The listing builds one solid part. Answer for the finished solid, in the listing's coordinates (mm). A direction names the side the tool comes from. Coordinates: 2 decimals unless noted, no trailing zeros. Loops run counter-clockwise (first coordinate to the right, second up) from the corner with the lowest first, then second, coordinate; pieces in that order, holes last. Notation, with made-up numbers: (-26.5, 74.5) - (-20.5, 74.5) arc R19 ccw to (-20.5, 100.5) - close; hole circle Ø6 at (-37, 14). An arc over 180 degrees is marked (long way). Use one line per item in the form item = value. Start each with the question number.
```python
from build123d import *

# Parameters (mm, degrees)
F0_W      = 117.213294
F0_H      = 67.42356
F1_DEPTH  = 25.4
F1_FACE_W = 117.213294
F1_FACE_H = 67.42356
F2_DEPTH  = 12.7
F3_R      = 45.862113
F3_R_2    = 37.681332
F4_DEPTH  = 63.5
F5_W      = 74.026364
F5_H      = 21.373598
F6_DEPTH  = 50.8
F8_DEPTH  = 25.4


with BuildPart() as f1:
    # F0 (on Top) → F1 (new body)
    with BuildSketch(Plane.XY):
        with Locations((9.024359, -5.497601)):
            Rectangle(F0_W, F0_H)
    extrude(amount=F1_DEPTH)

    # F1_face (on face) → F2 (cut)
    with BuildSketch(Plane(origin=(9.024359, -5.497601, 25.4), x_dir=(1, 0, 0), z_dir=(0, 0, 1))):
        Rectangle(F1_FACE_W, F1_FACE_H)
    extrude(amount=-F2_DEPTH, mode=Mode.SUBTRACT)

    # F3 (on Top) → F4 (join)
    with BuildSketch(Plane.XY):
        with Locations((96.162871, -7.875698)):
            Circle(F3_R)
        with Locations((96.162871, -7.875698)):
            Circle(F3_R_2, mode=Mode.SUBTRACT)
    extrude(amount=F4_DEPTH)

    # F5 (on face) → F6 (join)
    with BuildSketch(Plane.XY.offset(12.7)):
        with Locations((15.318876, -10.686799)):
            Rectangle(F5_W, F5_H)
    extrude(amount=F6_DEPTH)

    # F7 (on face) → F8 (cut)
    with BuildSketch(Plane.XZ.offset(21.373598)):
        Polygon((-21.694306, 63.5), (-21.694306, 12.7), (52.332058, 63.5), align=None)
    extrude(amount=-F8_DEPTH, mode=Mode.SUBTRACT)


solid = f1.part
```
(1) A cutting plane is placed at B-B (x = 127). Determine the outline of the cut face in (y, z).
(2) Each of these flat-tipped pins is pushed along its axis until it touches: pin 1 Ø10 at (x, z) = (27, 8.5) entering from +Y; pin 2 Ø4 at (y, z) = (22.5, 53) entering from -X; pin 3 Ø12 at (x, z) = (29.5, 38) entering from -Y; pin 4 Ø10 at (x, y) = (91.5, 22) entering from -Z. Where does it stop, or does it pass through?
(3) Find the intervals of material crossed by probe 1 along Y at (x, z) = (96.5, 33.5); probe 2 along Y at (x, z) = (21, 38); probe 3 along Z at (x, y) = (60.5, -12.5), in increasing order. Write a range as from..to.
(4) A cutting plane is placed at D-D (x = 13.5). Determine the outline of the cut face in (y, z).
(5) Determine the mould class of faces 4 (the face through (8, 28.214, 6)), 5 (the face through (24, -7, 0)), 6 (the face through (132.104, 3.443, 31.306)) for opening direction Y: +Y half, -Y half, draft (parallel to the pull), parting line (faces both ways), or undercut.
(6) For faces 1 (the face through (30, 0, 26)), 2 (the face through (31, -21.374, 26)), 3 (the face through (67.631, -8, 6)), determine the directions among +Z, -Z, +X, -X, +Y, -Y from which every point of the face is accessible in a straight line to the end or side of a thin tool.
(7) A cutting plane is placed at A-A (y = -36). Determine the outline of the cut face in (x, z).
Evaluation:
q1.outline = (-41.82, 0) - (-29.53, 0) - (-29.53, 63.5) - (-41.82, 63.5) - close; (13.78, 0) - (26.07, 0) - (26.07, 63.5) - (13.78, 63.5) - close
q2.pin_1 = 28.21
q2.pin_2 = 60.13
q2.pin_3 = -21.37
q2.pin_4 = through
q3.probe_1 = -53.74..-45.56, 29.8..37.99
q3.probe_2 = -21.37..0
q3.probe_3 = 0..12.7
q4.outline = (-39.21, 0) - (28.21, 0) - (28.21, 12.7) - (0, 12.7) - (0, 36.85) - (-21.37, 36.85) - (-21.37, 12.7) - (-39.21, 12.7) - close
q5.face_4 = +Y half
q5.face_5 = draft
q5.face_6 = undercut
q6.face_1 = +Z, -X, +Y
q6.face_2 = +Z, -X, -Y
q6.face_3 = +Z, -Z
q7.outline = (-49.58, 0) - (71.08, 0) - (71.08, 63.5) - (59.94, 63.5) - (59.94, 12.7) - (-49.58, 12.7) - close; (121.24, 0) - (132.39, 0) - (132.39, 63.5) - (121.24, 63.5) - close
